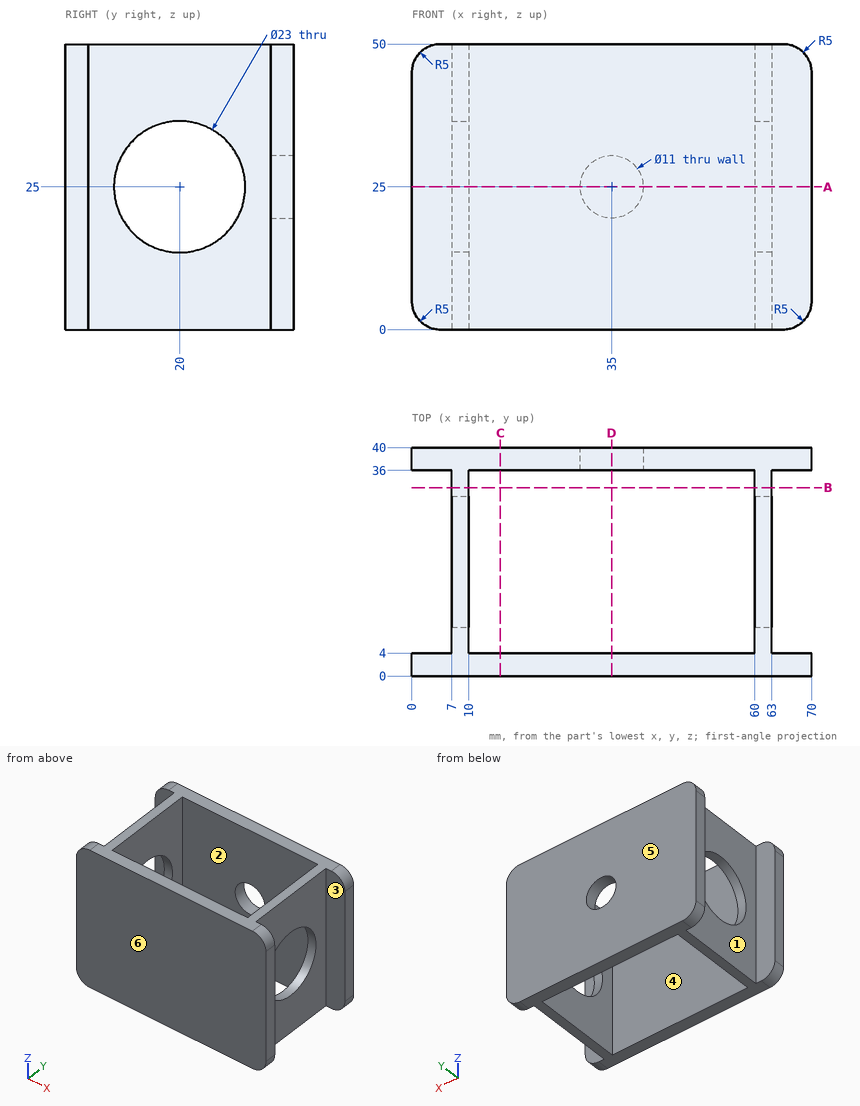
Print and shaded views of the part. All mm, measured from the part's lowest x, y and z. A direction names the side the tool comes from. Coordinates: 2 decimals unless noted, no trailing zeros. Order: outer loops, then holes, each group sorted by start corner. A loop starts at its lowest first (then second) coordinate and runs counter-clockwise, first axis right, second up.
Item 1: Drill centre lines: L1, parallel to Y at x = 65.5, z = 40; L2, parallel to X at y = 31, z = 15.5; L3, parallel to Y at x = 61, z = 25. Where is each one in solid material? Low to high.
Filled in:
L1: y = 0 to 4, 36 to 40
L2: x = 7 to 10, 60 to 63
L3: y = 0 to 8.5, 31.5 to 40
Item 2: Drop flat-ended pins along their axis: pin 1 Ø16 at (y, z) = (15.5, 24.5) entering from -X; pin 2 Ø12 at (y, z) = (14, 13) entering from +X. Give the stop position or say it passes through.
Filled in:
pin 1: stops at x = 7
pin 2: stops at x = 63
Item 3: Saw through at D-D on x = 35. List the corners of the cut face in (y, z), then the cut area to 3 significant figures.
Filled in:
outline: (0, 0) - (4, 0) - (4, 50) - (0, 50) - close; (36, 0) - (40, 0) - (40, 19.5) - (36, 19.5) - close; (36, 30.5) - (40, 30.5) - (40, 50) - (36, 50) - close
area: 356 mm2
Item 4: Saw through at A-A on z = 25. List the corners of the cut face in (x, y).
Filled in:
outline: (0, 0) - (70, 0) - (70, 4) - (63, 4) - (63, 8.5) - (60, 8.5) - (60, 4) - (10, 4) - (10, 8.5) - (7, 8.5) - (7, 4) - (0, 4) - close; (0, 36) - (7, 36) - (7, 31.5) - (10, 31.5) - (10, 36) - (29.5, 36) - (29.5, 40) - (0, 40) - close; (40.5, 36) - (60, 36) - (60, 31.5) - (63, 31.5) - (63, 36) - (70, 36) - (70, 40) - (40.5, 40) - close
Item 5: Mould opens along Y. For the marked faces 4, 5 and 6 say: released by +Y, released by -Y, zero draft, split by the parting line, or undercut.
Filled in:
face 4: undercut
face 5: released by +Y
face 6: released by -Y
Item 6: Saw through at B-B on y = 33. List the corners of the cut face in (x, z).
Filled in:
outline: (7, 0) - (10, 0) - (10, 50) - (7, 50) - close; (60, 0) - (63, 0) - (63, 50) - (60, 50) - close
Item 7: Saw through at C-C on x = 15.5. List the corners of the cut face in (y, z).
Filled in:
outline: (0, 0) - (4, 0) - (4, 50) - (0, 50) - close; (36, 0) - (40, 0) - (40, 50) - (36, 50) - close
Item 8: Tool access for the marked faces 1, 2 and 3: list every direction of +Z, -Z, +X, -X, +Y, -Y with a clear straight run to the whole face (end or side of a thin tool).
Filled in:
face 1: +Z, -Z, -X
face 2: +Z, -Z
face 3: +Z, -Z, +X
